```python
from build123d import *

# Parameters (mm, degrees)
BOSS_EXTRUDE3_DEPTH = 5
SKETCH6_R           = 5
CUT_EXTRUDE1_DEPTH  = 6


with BuildPart() as part:
    # Sketch4 → Boss-Extrude3 (new body)
    with BuildSketch(Plane.XY):
        with BuildLine():
            Line((-25, -290), (25, -290))
            ThreePointArc((25, -290), (32.071067812, -287.071067812), (35, -280))
            Line((35, -280), (35, -10))
            ThreePointArc((35, -10), (32.071067812, -2.928932188), (25, 0))
            Line((25, 0), (-25, 0))
            ThreePointArc((-25, 0), (-32.071067812, -2.928932188), (-35, -10))
            Line((-35, -10), (-35, -280))
            ThreePointArc((-35, -280), (-32.071067812, -287.071067812), (-25, -290))
        make_face()
    extrude(amount=BOSS_EXTRUDE3_DEPTH)

    # Sketch6 → Cut-Extrude1 (cut, through all)
    with BuildSketch(Plane.XY.offset(5)):
        with Locations((0, -9)):
            Circle(SKETCH6_R)
        with BuildLine():
            Line((-17.5, -20), (17.5, -20))
            ThreePointArc((17.5, -20), (21.035533906, -21.464466094), (22.5, -25))
            Line((22.5, -25), (22.5, -280))
            ThreePointArc((22.5, -280), (21.035533906, -283.535533906), (17.5, -285))
            Line((17.5, -285), (-17.5, -285))
            ThreePointArc((-17.5, -285), (-21.035533906, -283.535533906), (-22.5, -280))
            Line((-22.5, -280), (-22.5, -25))
            ThreePointArc((-22.5, -25), (-21.035533906, -21.464466094), (-17.5, -20))
        make_face()
    extrude(amount=-CUT_EXTRUDE1_DEPTH, mode=Mode.SUBTRACT)


solid = part.part
```
Source: CAD feature listing. Evaluate the final solid. Frame: model axes, mm. A direction names the side the tool comes from. Round coordinates to 2 decimals unless told otherwise and drop trailing zeros. Loops run counter-clockwise (first coordinate to the right, second up) from the corner with the lowest first, then second, coordinate; pieces in that order, holes last. Notation, with made-up numbers: (-7.75, 17.5) - (50.25, 17.5) arc R17 cw to (50.25, 35.5) - close; hole circle Ø8 at (-38.5, 71.5). An arc over 180 degrees is marked (long way). Use CSV: the item, a comma, the result in double quotes.
Q1. Mould query, pull axis Y, two halves, no side actions, for faces 3 (the cylindrical face through (21.07, -283.5, 2.54)), 4 (the flat face through (0, -20, 3)), 5 (the cylindrical face through (32.15, -3.01, 2.46)), 6 (the cylindrical face through (-32.15, -286.99, 2.46)). Classes: pulls with the +Y half, pulls with the -Y half, needs draft (parallel to the pull), parting line crosses it, or undercut.
Reported:
face 3,"undercut"
face 4,"undercut"
face 5,"pulls with the +Y half"
face 6,"pulls with the -Y half"
Q2. Section query A-A, the plane x = 8.5. Output: boundary loops of the cut face in (y, z), then the cut area to 3 significant figures.
Reported:
outline,"(-290, 0) - (-285, 0) - (-285, 5) - (-290, 5) - close; (-20, 0) - (0, 0) - (0, 5) - (-20, 5) - close"
area,"125 mm^2"
Q3. Ray query, line 1 along Y through (x, z) = (0, 1.35); line 2 along Y through (x, z) = (11, 3.05); line 3 along X through (y, z) = (-219, 4.45). Return the intervals inside material, ascending.
Reported:
line 1,"-290 to -285, -20 to -14, -4 to 0"
line 2,"-290 to -285, -20 to 0"
line 3,"-35 to -22.5, 22.5 to 35"
Q4. Section query C-C, the plane z = 1.7. Output: boundary loops of the cut face in (x, y).
Reported:
outline,"(-35, -280) arc R10 ccw to (-25, -290) - (25, -290) arc R10 ccw to (35, -280) - (35, -10) arc R10 ccw to (25, 0) - (-25, 0) arc R10 ccw to (-35, -10) - close; hole (-22.5, -280) arc R5 ccw to (-17.5, -285) - (17.5, -285) arc R5 ccw to (22.5, -280) - (22.5, -25) arc R5 ccw to (17.5, -20) - (-17.5, -20) arc R5 ccw to (-22.5, -25) - close; hole circle Ø10 at (0, -9)"
Q5. Reachability of faces 1 (the flat face through (-35, -143, 2)), 2 (the cylindrical face through (-21, -283.57, 2.54)) from +Z, -Z, +X, -X, +Y, -Y: full face, straight path, thin tool, end or side. Return the list, or none.
Reported:
face 1,"+Z, -Z, -X, +Y, -Y"
face 2,"+Z, -Z"
Q6. Pin query (flat end, axial travel): pin 1 Ø16 at (x, y) = (0, -9) entering from +Z. Return the tip coordinate at first contact, or that it passes through.
Reported:
pin 1,"z = 5"
Q7. Section query B-B, the plane y = -200.5. Output: boundary loops of the cut face in (x, z).
Reported:
outline,"(-35, 0) - (-22.5, 0) - (-22.5, 5) - (-35, 5) - close; (22.5, 0) - (35, 0) - (35, 5) - (22.5, 5) - close"
